Work out the finished part from the listing and answer in its coordinate system (mm). Face numbers are marked on the shaded views. A direction names the side the tool comes from. Give positions to 0.01 mm unless a question says otherwise; leave off trailing zeros. Order: outer loops, then holes, each group sorted by start corner. A loop starts at its lowest first (then second) coordinate and runs counter-clockwise, first axis right, second up. Notation, with made-up numbers: (-10, -19) - (-3, -19) arc R11 ccw to (-3, -9) - close; hole circle Ø7 at (4, 60.25). An arc over 180 degrees is marked (long way). Return JSON: item names as keys, results as strings. Group by question number.
from build123d import *

# Parameters (mm, degrees)
SKETCH1_R            = 22.225
SKETCH1_R_2          = 15.24
BOSS_EXTRUDE1_DEPTH  = 5.08
SKETCH6_W            = 64.917410467
SKETCH6_H            = 82.171101747
CUT_EXTRUDE2_DEPTH   = 32.838775887
BOSS_EXTRUDE3_DEPTH  = 5.08
MIRROR2_COPY_1_DEPTH = 5.08
FILLET5_R            = 2.54
SKETCH15_W           = 12.7
SKETCH15_H           = 4.7625
BOSS_EXTRUDE5_DEPTH  = 14.732
SKETCH17_R           = 2.15265
CUT_EXTRUDE5_DEPTH   = 12.7
FILLET6_R            = 6.35
FILLET6_OF_MIRROR3_R = 6.35


with BuildPart() as part:
    # Sketch1 → Boss-Extrude1 (new body)
    with BuildSketch(Plane(origin=(0, 0, 0), x_dir=(1, 0, 0), z_dir=(0, 1, 0))):
        with Locations(Location((0, 0, 0), (0, 0, 270))):
            Circle(SKETCH1_R)
        with Locations(Location((0, 0, 0), (0, 0, 270))):
            Circle(SKETCH1_R_2, mode=Mode.SUBTRACT)
    boss_extrude1 = extrude(amount=BOSS_EXTRUDE1_DEPTH)

    # Sketch6 → Cut-Extrude2 (cut, through all)
    with BuildSketch(Plane(origin=(0, 5.08, 0), x_dir=(1, 0, 0), z_dir=(0, 1, 0))):
        with Locations((-24.203705233, -1.153387837)):
            Rectangle(SKETCH6_W, SKETCH6_H)
    cut_extrude2 = extrude(amount=-CUT_EXTRUDE2_DEPTH, mode=Mode.SUBTRACT)

    # Sketch9 → Boss-Extrude3 (add)
    with BuildSketch(Plane(origin=(0, 5.08, 0), x_dir=(1, 0, 0), z_dir=(0, 1, 0))):
        Polygon((8.255, 20.635057548), (8.255, 46.035057548), (14.605, 46.035057548), (14.605, 16.752450567), align=None)
    boss_extrude3 = extrude(amount=-BOSS_EXTRUDE3_DEPTH)

    # Mirror1: Boss-Extrude3 across plane
    add(boss_extrude3.mirror(Plane.XY))

    # Mirror2: Boss-Extrude1, Cut-Extrude2, Boss-Extrude3 across plane
    add(boss_extrude1.mirror(Plane.ZX))
    add(cut_extrude2.mirror(Plane.ZX), mode=Mode.SUBTRACT)
    add(boss_extrude3.mirror(Plane.ZX))

    # Mirror2 copy 1 sketch → Mirror2 copy 1 (add)
    with BuildSketch(Plane.XZ.offset(5.08)):
        Polygon((8.255, 20.635057548), (8.255, 46.035057548), (14.605, 46.035057548), (14.605, 16.752450567), align=None)
    extrude(amount=-MIRROR2_COPY_1_DEPTH)

    # Fillet5
    fillet5_edges = [part.edges().sort_by_distance(p)[0] for p in [
        (11.43, -5.08, -46.035057548),
        (11.43, -5.08, 46.035057548),
        (11.43, 5.08, -46.035057548),
        (8.255, 0, -46.035057548),
        (14.605, 0, -46.035057548),
        (11.43, 5.08, 46.035057548),
        (14.605, 0, 46.035057548),
        (8.255, 0, 46.035057548),
    ]]
    fillet(fillet5_edges, radius=FILLET5_R)

    # Sketch15 → Boss-Extrude5 (add)
    with BuildSketch(Plane.ZY.offset(-8.255)):
        with Locations((-37.145057548, 2.69875)):
            Rectangle(SKETCH15_W, SKETCH15_H)
    boss_extrude5 = extrude(amount=BOSS_EXTRUDE5_DEPTH)

    # Sketch17 → Cut-Extrude5 (cut)
    with BuildSketch(Plane(origin=(0, 5.08, 0), x_dir=(1, 0, 0), z_dir=(0, 1, 0))):
        with Locations(Location((-0.127, 37.084, 0), (0, 0, 270))):
            Circle(SKETCH17_R)
    cut_extrude5 = extrude(amount=-CUT_EXTRUDE5_DEPTH, mode=Mode.SUBTRACT)

    # Fillet6
    fillet6_edges = [part.edges().sort_by_distance(p)[0] for p in [
        (8.255, 2.69875, -30.795057548),
        (-6.477, 2.69875, -30.795057548),
        (-6.477, 2.69875, -43.495057548),
    ]]
    fillet(fillet6_edges, radius=FILLET6_R - 0.0001)  # a hair under: the kernel refuses the full size

    # Mirror3: Boss-Extrude5, Cut-Extrude5 across plane
    add(boss_extrude5.mirror(Plane.XY))
    add(cut_extrude5.mirror(Plane.XY), mode=Mode.SUBTRACT)

    # Fillet6 of Mirror3
    fillet6_of_mirror3_edges = [part.edges().sort_by_distance(p)[0] for p in [
        (8.255, 2.69875, 30.795057548),
        (-6.477, 2.69875, 30.795057548),
        (-6.477, 2.69875, 43.495057548),
    ]]
    fillet(fillet6_of_mirror3_edges, radius=FILLET6_OF_MIRROR3_R - 0.0001)  # a hair under: the kernel refuses the full size


solid = part.part
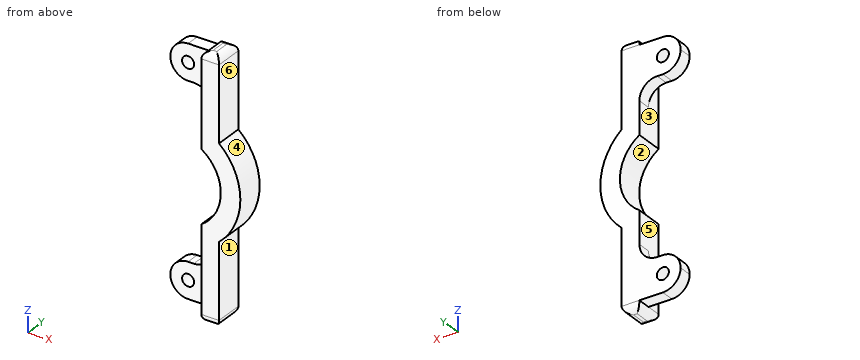
1. The part is cut by section C-C (y = 3.5). State how many separate pieces and enclosed holes the cut face has, and give its area (3 significant figures).
2. The part is cut by section B-B (y = -0.5). Give the vertices of the cut face in (x, z) (3 decimals).
3. Consider probe 1 along Y at (x, z) = (7, -32); probe 2 along Z at (x, y) = (-1.5, 2.25); probe 3 along X at (y, z) = (-0.25, 31) (3 decimals). Determine where each line is inside the solid, lowest interval first. Write a range as from..to.
4. The part is cut by section A-A (x = 5). Give the vertices of the cut face in (y, z).
5. Determine the mould class of the marked faces 3, 4, 5 and 6 for opening direction Z: released by +Z, released by -Z, zero draft, split by the parting line, or undercut.
6. Each of these flat-tipped pins is pushed along its axis until it touches: pin 1 (16 mm diameter, centred on x = -1, z = -36, fed in from -Y); pin 2 (4 mm diameter, centred on y = -2, z = -10, fed in from -X); pin 3 (5 mm diameter, centred on y = -2, z = 33, fed in from -X); pin 4 (2.5 mm diameter, centred on x = -0.127, z = 37.084, fed in from -Y). Where does it stop, or does it pass through?
7. A tool of negligible diameter and unlimited length cuts with its end or side. For the marked faces 1 and 2, from which of +Z, -Z, +X, -X, +Y, -Y can it reach the whole face along a straight path? Write none if from no direction.
Answers:
{
 "1": {"separate pieces": "1", "enclosed holes": "2", "area": "957 mm^2"},
 "2": {"outline": "(8.255, -43.495) arc R2.54 ccw to (10.795, -46.035) - (12.065, -46.035) arc R2.54 ccw to (14.605, -43.495) - (14.605, -16.752) arc R22.225 ccw to (14.605, 16.752) - (14.605, 43.495) arc R2.54 ccw to (12.065, 46.035) - (10.795, 46.035) arc R2.54 ccw to (8.255, 43.495) - (8.255, 12.811) arc R15.24 cw to (8.255, -12.811) - close"},
 "3": {"probe 1": "y = 0.32..5.08", "probe 2": "z = -43.34..-38.74, -35.43..-30.95, 30.95..35.43, 38.74..43.34", "probe 3": "x = 8.255..14.605"},
 "4": {"outline": "(0.32, -43.5) - (5.08, -43.5) - (5.08, -29.99) - (0.32, -29.99) - close; (0.32, 29.99) - (5.08, 29.99) - (5.08, 43.5) - (0.32, 43.5) - close"},
 "5": {"face 3": "undercut", "face 4": "split by the parting line", "face 5": "undercut", "face 6": "zero draft"},
 "6": {"pin 1": "stops at y = 0.32", "pin 2": "stops at x = 9.39", "pin 3": "stops at x = -5.61", "pin 4": "passes through"},
 "7": {"face 1": "-Z, +X, +Y, -Y", "face 2": "-X, +Y, -Y"}
}
